from build123d import *

# Parameters (mm, degrees)
SKETCH1_W                = 177.8
SKETCH1_H                = 177.8
SKETCH1_W_2              = 159.078855478
SKETCH1_H_2              = 159.078855478
BOSS_EXTRUDE1_DEPTH      = 38.1
BOSS_EXTRUDE1_DEPTH_BACK = 59.182
BOSS_EXTRUDE3_START      = 38.1
SKETCH1_5_W              = 177.8
SKETCH1_5_H              = 177.8
SKETCH1_5_W_2            = 159.078855478
SKETCH1_5_H_2            = 159.078855478
SKETCH1_5_R              = 11.43
BOSS_EXTRUDE3_DEPTH      = 5.08
FILLET1_R                = 5.08
SKETCH3_R                = 1.7
CUT_EXTRUDE1_DEPTH       = 103.362
FILLET2_R                = 2.54
SKETCH4_R                = 2.05
CUT_EXTRUDE2_DEPTH       = 5.08
SKETCH5_W                = 28.575
SKETCH5_H                = 12.7
CUT_EXTRUDE3_DEPTH       = 9.360572


with BuildPart() as part:
    # Sketch1 → Boss-Extrude1 (new body, two sides)
    with BuildSketch(Plane(origin=(0, 0, 0), x_dir=(1, 0, 0), z_dir=(0, 1, 0))) as boss_extrude1_sk:
        Rectangle(SKETCH1_W, SKETCH1_H)
        Rectangle(SKETCH1_W_2, SKETCH1_H_2, mode=Mode.SUBTRACT)
    extrude(amount=BOSS_EXTRUDE1_DEPTH)
    extrude(boss_extrude1_sk.sketch, amount=-BOSS_EXTRUDE1_DEPTH_BACK)

    # Sketch1<5> → Boss-Extrude3 (add)
    with BuildSketch(Plane(origin=(0, 0, 0), x_dir=(1, 0, 0), z_dir=(0, 1, 0)).offset(BOSS_EXTRUDE3_START)):
        Rectangle(SKETCH1_5_W, SKETCH1_5_H)
        Rectangle(SKETCH1_5_W_2, SKETCH1_5_H_2, mode=Mode.SUBTRACT)
        Rectangle(SKETCH1_5_W_2, SKETCH1_5_H_2)
        Circle(SKETCH1_5_R, mode=Mode.SUBTRACT)
    extrude(amount=BOSS_EXTRUDE3_DEPTH)

    # Fillet1
    fillet1_edges = [part.edges().sort_by_distance(p)[0] for p in [
        (-88.9, -8.001, 88.9),
        (-88.9, -8.001, -88.9),
        (88.9, -8.001, -88.9),
        (88.9, -8.001, 88.9),
    ]]
    fillet(fillet1_edges, radius=FILLET1_R)

    # Sketch3 → Cut-Extrude1 (cut, through all)
    with BuildSketch(Plane(origin=(0, 43.18, 0), x_dir=(1, 0, 0), z_dir=(0, 1, 0))):
        with Locations((-15.5, 15.5)):
            Circle(SKETCH3_R)
        with Locations((-15.5, -15.5)):
            Circle(SKETCH3_R)
        with Locations((15.5, 15.5)):
            Circle(SKETCH3_R)
        with Locations((15.5, -15.5)):
            Circle(SKETCH3_R)
    extrude(amount=-CUT_EXTRUDE1_DEPTH, mode=Mode.SUBTRACT)

    # Fillet2
    fillet2_edges = [part.edges().sort_by_distance(p)[0] for p in [
        (79.539427739, -10.541, -79.539427739),
        (-79.539427739, -10.541, -79.539427739),
        (-79.539427739, -10.541, 79.539427739),
        (79.539427739, -10.541, 79.539427739),
    ]]
    fillet(fillet2_edges, radius=FILLET2_R)

    # Sketch4 → Cut-Extrude2 (cut)
    with BuildSketch(Plane(origin=(0, 43.18, 0), x_dir=(1, 0, 0), z_dir=(0, 1, 0))):
        with Locations((-40.66, 40.66)):
            Circle(SKETCH4_R)
        with Locations((40.66, 40.66)):
            Circle(SKETCH4_R)
        with Locations((-40.66, -40.66)):
            Circle(SKETCH4_R)
        with Locations((40.66, -40.66)):
            Circle(SKETCH4_R)
    extrude(amount=-CUT_EXTRUDE2_DEPTH, mode=Mode.SUBTRACT)

    # Sketch5 → Cut-Extrude3 (cut)
    with BuildSketch(Plane.XY.offset(88.9)):
        with Locations((-57.223240987, -41.174341157)):
            Rectangle(SKETCH5_W, SKETCH5_H)
    extrude(amount=-CUT_EXTRUDE3_DEPTH, mode=Mode.SUBTRACT)


solid = part.part
Read the model definition and answer for the solid it produces. Units are mm, in the model's axes. A direction names the side the tool comes from. Give positions to 0.01 mm unless a question says otherwise; leave off trailing zeros. Write each loop counter-clockwise with the first axis right and the second up, starting at its lowest first coordinate (ties: lowest second). Pieces come first, ordered by that corner, then holes. Notation, with made-up numbers: (53, 88.25) - (90, 88.25) arc R16 cw to (90, 93.25) - close; hole circle Ø4 at (28.25, -16.75). An arc over 180 degrees is marked (long way). Return JSON: item names as keys, results as strings.
Q1. A cutting plane is placed at D-D, the plane z = -63. Determine the outline of the cut face in (x, y).
Reply:
{"outline": "(-88.9, -59.18) - (-79.54, -59.18) - (-79.54, 38.1) - (79.54, 38.1) - (79.54, -59.18) - (88.9, -59.18) - (88.9, 43.18) - (-88.9, 43.18) - close"}
Q2. For faces 1 (the face through (-1, 38.1, -19)), 2 (the face through (-87.451, -8.718, -87.372)), 3 (the face through (-42.936, -41, 84)), determine the directions among +Z, -Z, +X, -X, +Y, -Y from which every point of the face is accessible in a straight line to the end or side of a thin tool.
Reply:
{"face 1": "-Y", "face 2": "-Z, -X, +Y, -Y", "face 3": "+Z"}
Q3. Consider line 1 along X through (y, z) = (39.35, 15.5); line 2 along X through (y, z) = (39.95, 40.66). Determine where each line is inside the solid, lowest interval first. Write a range as [from, to].
Reply:
{"line 1": "[-88.9, -17.2], [-13.8, 13.8], [17.2, 88.9]", "line 2": "[-88.9, -42.71], [-38.61, 38.61], [42.71, 88.9]"}
Q4. A cutting plane is placed at B-B, the plane x = 7.5. Determine the outline of the cut face in (y, z).
Reply:
{"outline": "(-59.18, -88.9) - (43.18, -88.9) - (43.18, -8.63) - (38.1, -8.63) - (38.1, -79.54) - (-59.18, -79.54) - close; (-59.18, 79.54) - (38.1, 79.54) - (38.1, 8.63) - (43.18, 8.63) - (43.18, 88.9) - (-59.18, 88.9) - close"}
Q5. A cutting plane is placed at A-A, the plane z = 0. Determine the outline of the cut face in (x, y).
Reply:
{"outline": "(-88.9, -59.18) - (-79.54, -59.18) - (-79.54, 38.1) - (-11.43, 38.1) - (-11.43, 43.18) - (-88.9, 43.18) - close; (11.43, 38.1) - (79.54, 38.1) - (79.54, -59.18) - (88.9, -59.18) - (88.9, 43.18) - (11.43, 43.18) - close"}
Q6. A cutting plane is placed at C-C, the plane y = -42. Determine the outline of the cut face in (x, z), and give its area (3 significant figures).
Reply:
{"outline": "(-88.9, -83.82) arc R5.08 ccw to (-83.82, -88.9) - (83.82, -88.9) arc R5.08 ccw to (88.9, -83.82) - (88.9, 83.82) arc R5.08 ccw to (83.82, 88.9) - (-42.94, 88.9) - (-42.94, 79.54) - (77, 79.54) arc R2.54 cw to (79.54, 77) - (79.54, -77) arc R2.54 cw to (77, -79.54) - (-77, -79.54) arc R2.54 cw to (-79.54, -77) - (-79.54, 77) arc R2.54 cw to (-77, 79.54) - (-71.51, 79.54) - (-71.51, 88.9) - (-83.82, 88.9) arc R5.08 ccw to (-88.9, 83.82) - close", "area": "6,020 mm²"}
Q7. For a pull along Z with two mould halves and no side action, classify faces 4 (the face through (79.539, -10, 1)), 5 (the face through (-1, -9, 88.9)), 6 (the face through (-71.511, -41, 84)) as released by +Z, released by -Z, zero draft, split by the parting line, or undercut.
Reply:
{"face 4": "undercut", "face 5": "released by +Z", "face 6": "zero draft"}
Q8. Given P1, Ø3, axis at y = -40, z = 85, coming from the +X side; P2, Ø12, axis at x = -44.5, z = 64, coming from the -Y side, each flat-ended and moving along its own axis, determine where each tip first touches the part or whether it passes through.
Reply:
{"P1": "x = 88.9", "P2": "y = 38.1"}
